The listing builds one solid part. Answer for the finished solid, in the listing's coordinates (mm). Face numbers are marked on the shaded views. A direction names the side the tool comes from. Give positions to 0.01 mm unless a question says otherwise; leave off trailing zeros. Write each loop counter-clockwise with the first axis right and the second up, starting at its lowest first coordinate (ties: lowest second). Pieces come first, ordered by that corner, then holes. Notation, with made-up numbers: (66, 68.25) - (125, 68.25) arc R29 cw to (125, 100.25) - close; hole circle Ø1 at (38.25, 68). An arc over 180 degrees is marked (long way). Answer as CSV lines item,"result". Start each with the question number.
(1) Find section C-C (z = 1). Write down the section's boundary in (x, y), then the cut area to 3 significant figures.
(2) For the marked faces 1, 2, 3, 4 and 5, determine the directions among +Z, -Z, +X, -X, +Y, -Y from which every point of the face is accessible in a straight line to the end or side of a thin tool.
(3) Find section D-D (x = -8.5). Write down the section's boundary in (y, z), then the cut area to 4 significant figures.
(4) Each of these flat-tipped pins is pushed along its axis until it touches: pin 1 Ø2.5 at (x, z) = (23.5, 9.5) entering from -Y; pin 2 Ø10 at (x, y) = (5, -3.5) entering from +Z; pin 3 Ø4 at (x, y) = (4, -23.5) entering from +Z. Where does it stop, or does it pass through?
(5) For a pull along X with two mould halves and no side action, classify the marked faces 6, 7 and 8 as pulls with the +X half, pulls with the -X half, needs draft (parallel to the pull), parting line crosses it, or undercut.
(6) Find section A-A (x = 0). Write down the section's boundary in (y, z), then the cut area to 3 significant figures.
(7) Straight lines are drawn through the part: probe 1 along X at (y, z) = (-24.75, 2.75); probe 2 along X at (y, z) = (-5, 0.8); probe 3 along X at (y, z) = (-21.75, 10). For each, find the intervals that lie inside material, in ascending order.
(8) Find section B-B (y = -23.25). Write down the section's boundary in (x, z).
from build123d import *

# Parameters (mm, degrees)
SKETCH_R        = 2.5
PAD_DEPTH       = 11
SKETCH001_W     = 93.08528
SKETCH001_H     = 10
POCKET_DEPTH    = 5
SKETCH002_W     = 55
SKETCH002_H     = 3
POCKET001_DEPTH = 13
POCKET002_DEPTH = 3.1
POCKET003_DEPTH = 5


with BuildPart() as part:
    # Sketch → Pad (new body)
    with BuildSketch(Plane.XY):
        Polygon((-29, 0), (29, 0), (32, -3), (32, -28), (18.85, -28), (18.85, -16.5), (2.35, -16.5), (2.35, -28), (-12.65, -28), (-12.65, -15), (-26.65, -15), (-26.65, -28), (-32, -28), (-32, -3), align=None)
        with Locations((0, -5)):
            Circle(SKETCH_R, mode=Mode.SUBTRACT)
    extrude(amount=PAD_DEPTH)

    # Sketch001 (on Face17 of Pad) → Pocket (cut)
    with BuildSketch(Plane.XY.offset(11)):
        with Locations((0, -5)):
            Rectangle(SKETCH001_W, SKETCH001_H)
    extrude(amount=-POCKET_DEPTH, mode=Mode.SUBTRACT)

    # Sketch002 (on Face11 of Pocket) → Pocket001 (cut)
    with BuildSketch(Plane.XZ.offset(28)):
        with Locations((0, 6.5)):
            Rectangle(SKETCH002_W, SKETCH002_H)
    extrude(amount=-POCKET001_DEPTH, mode=Mode.SUBTRACT)

    # Sketch003 (on Face4 of Pocket001) → Pocket002 (cut)
    with BuildSketch(Plane.XY.offset(6)):
        Polygon((3.983717, -5), (1.991858, -1.55), (-1.991858, -1.55), (-3.983717, -5), (-1.991858, -8.45), (1.991858, -8.45), align=None)
    extrude(amount=-POCKET002_DEPTH, mode=Mode.SUBTRACT)

    # Sketch004 (on Face25 of Pocket002) → Pocket003 (cut)
    with BuildSketch(Plane.XY.offset(11)):
        Polygon((-25.15, -5.838694), (-12.65, -5.838694), (-12.65, -16.5), (3.55, -16.5), (3.55, -5.838694), (18.55, -5.838694), (18.55, -16.5), (25.85, -16.5), (25.85, -33.515926), (-25.15, -33.515926), align=None)
    extrude(amount=-POCKET003_DEPTH, mode=Mode.SUBTRACT)


solid = part.part
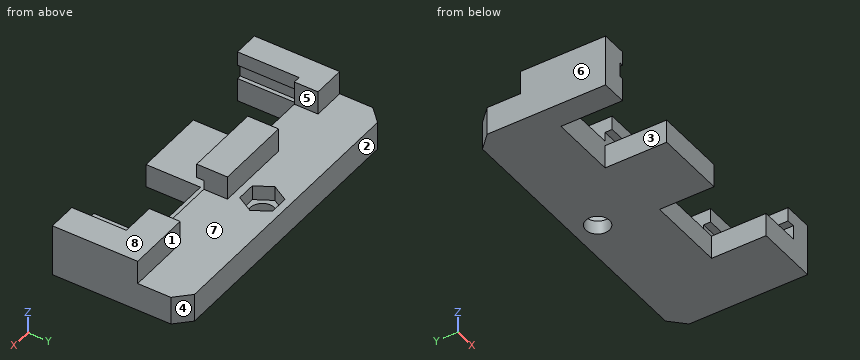
Result set:
1,outline,"(-32, -28) - (-26.65, -28) - (-26.65, -15) - (-12.65, -15) - (-12.65, -28) - (2.35, -28) - (2.35, -16.5) - (18.85, -16.5) - (18.85, -28) - (32, -28) - (32, -3) - (29, 0) - (-29, 0) - (-32, -3) - close; hole circle Ø5 at (0, -5)"
1,area,"1,390 mm^2"
2,face 1,"+Z, +X, -X, +Y"
2,face 2,"+Z, -Z, +X, -X, +Y"
2,face 3,"+Z, -Z, -Y"
2,face 4,"+Z, -Z, +X, +Y"
2,face 5,"+Z, +Y, -Y"
3,outline,"(-28, 0) - (0, 0) - (0, 6) - (-10, 6) - (-10, 11) - (-16.5, 11) - (-16.5, 8) - (-15, 8) - (-15, 5) - (-28, 5) - close"
3,area,"184.5 mm^2"
4,pin 1,"y = -16.5"
4,pin 2,"z = 6"
4,pin 3,"z = 5"
5,face 6,"pulls with the -X half"
5,face 7,"undercut"
5,face 8,"needs draft"
6,outline,"(-28, 0) - (-7.5, 0) - (-7.5, 2.9) - (-8.45, 2.9) - (-8.45, 6) - (-10, 6) - (-10, 11) - (-16.5, 11) - (-16.5, 8) - (-15, 8) - (-15, 5) - (-28, 5) - close; (-2.5, 0) - (0, 0) - (0, 6) - (-1.55, 6) - (-1.55, 2.9) - (-2.5, 2.9) - close"
6,area,"149 mm^2"
7,probe 1,"-32 to -26.65, -12.65 to 2.35, 18.85 to 32"
7,probe 2,"-32 to -2.5, 2.5 to 32"
7,probe 3,"-32 to -26.65, 25.85 to 32"
8,outline,"(-32, 0) - (-26.65, 0) - (-26.65, 5) - (-27.5, 5) - (-27.5, 8) - (-26.65, 8) - (-26.65, 11) - (-32, 11) - close; (-12.65, 0) - (2.35, 0) - (2.35, 5) - (-12.65, 5) - close; (18.85, 0) - (32, 0) - (32, 11) - (25.85, 11) - (25.85, 8) - (27.5, 8) - (27.5, 5) - (18.85, 5) - close"
